from build123d import *

# Parameters (mm, degrees)
F0_R     = 360
F0_R_2   = 270
F1_DEPTH = 180
F2_SIZE  = 20
F3_SIZE  = 20


with BuildPart() as f1:
    # F0 (on Front) → F1 (new body, symmetric)
    with BuildSketch(Plane.XZ):
        Circle(F0_R)
        Circle(F0_R_2, mode=Mode.SUBTRACT)
    extrude(amount=F1_DEPTH, both=True)

    # F2
    f2_edges = [f1.edges().sort_by_distance(p)[0] for p in [
        (-360, -180, 0),
    ]]
    chamfer(f2_edges, length=F2_SIZE)

    # F3
    f3_edges = [f1.edges().sort_by_distance(p)[0] for p in [
        (-360, 180, 0),
    ]]
    chamfer(f3_edges, length=F3_SIZE)


solid = f1.part
Could you check a few things on this model? Use its own coordinates, in mm. Give positions to 0.01 mm unless a question says otherwise; leave off trailing zeros. Loops run counter-clockwise (first coordinate to the right, second up) from the corner with the lowest first, then second, coordinate; pieces in that order, holes last. Notation, with made-up numbers: (-5.5, -20) -> (29.5, -20) arc R22 ccw to (29.5, 9) -> close; hole circle Ø10 at (-9.5, 52). An arc over 180 degrees is marked (long way). Answer as CSV lines item,"result". Start each with the question number.
(1) If we section it at B-B on z = 0: Write out the boundary of the cut face in (x, y).
(2) If we section it at C-C on y = -115: Write out the boundary of the cut face in (x, z), then the cut area to 3 significant figures.
(3) If we section it at A-A on x = 0: Write out the boundary of the cut face in (y, z).
(4) I'm going to push flat-ended pins straight in: pin 1 Ø10 at (x, y) = (-257.5, 94.5) entering from +Z; pin 2 Ø3 at (x, y) = (144, 58.5) entering from +Z; pin 3 Ø10 at (y, z) = (-71, 246.5) entering from -X. Where does each tip first touch, or does it pass through?
(5) We'd pull the mould along Z, two halves only. Please class faces 1 (the conical face through (-44.39, 179.03, 338.07)), 2 (the flat face through (99, -180, 253)), 3 (the cylindrical face through (-214.263, 2.52, -164.291)): released by +Z, released by -Z, zero draft, split by the parting line, or undercut.
(6) I need wall thicknesses on probe 1 along Z at (x, y) = (0, 17); probe 2 along X at (y, z) = (-132, -193.5); probe 3 along Z at (x, y) = (157.5, -121.5). Which ranges of each line are inside material? Lowest first, please.
Computed:
1,outline,"(-360, -160) -> (-340, -180) -> (-270, -180) -> (-270, 180) -> (-340, 180) -> (-360, 160) -> close; (270, -180) -> (340, -180) -> (360, -160) -> (360, 160) -> (340, 180) -> (270, 180) -> close"
2,outline,"circle Ø720 at (0, 0); hole circle Ø540 at (0, 0)"
2,area,"178,000 mm2"
3,outline,"(-180, -340) -> (-160, -360) -> (160, -360) -> (180, -340) -> (180, -270) -> (-180, -270) -> close; (-180, 270) -> (180, 270) -> (180, 340) -> (160, 360) -> (-160, 360) -> (-180, 340) -> close"
4,pin 1,"stops at z = 256.6"
4,pin 2,"stops at z = 330.6"
4,pin 3,"stops at x = -266.98"
5,face 1,"split by the parting line"
5,face 2,"zero draft"
5,face 3,"undercut"
6,probe 1,"z = -360 to -270, 270 to 360"
6,probe 2,"x = -303.57 to -188.3, 188.3 to 303.57"
6,probe 3,"z = -323.72 to -219.3, 219.3 to 323.72"
